```python
from build123d import *

# Parameters (mm, degrees)
F0_W     = 170
F0_H     = 30
F1_DEPTH = 13
F3_DEPTH = 28
F4_W     = 110
F4_H     = 2
F5_DEPTH = 5
F6_SIZE  = 10
F7_R     = 5
F8_SIZE  = 1
F9_R     = 2


with BuildPart() as f1:
    # F0 (on Front) → F1 (new body)
    with BuildSketch(Plane.XZ):
        with Locations((0, 15)):
            Rectangle(F0_W, F0_H)
    extrude(amount=F1_DEPTH)

    # F2 (on face) → F3 (cut)
    with BuildSketch(Plane.XY.offset(30)):
        Polygon((-55, -2), (-71, -2), (-71, -12), (-65, -12), (-65, -13), (65, -13), (65, -12), (71, -12), (71, -2), (55, -2), (55, 0), (-55, 0), align=None)
    extrude(amount=-F3_DEPTH, mode=Mode.SUBTRACT)

    # F4 (on face) → F5 (join)
    with BuildSketch(Plane.XY.offset(2)):
        with Locations((0, -1)):
            Rectangle(F4_W, F4_H)
    extrude(amount=F5_DEPTH)

    # F6
    f6_edges = [f1.edges().sort_by_distance(p)[0] for p in [
        (85, -6.5, 0),
        (-85, -6.5, 0),
    ]]
    chamfer(f6_edges, length=F6_SIZE)

    # F7
    f7_edges = [f1.edges().sort_by_distance(p)[0] for p in [
        (-71, -7, 2),
        (71, -7, 2),
    ]]
    fillet(f7_edges, radius=F7_R)

    # F8
    f8_edges = [f1.edges().sort_by_distance(p)[0] for p in [
        (0, -13, 0),
        (0, 0, 0),
    ]]
    chamfer(f8_edges, length=F8_SIZE)

    # F9
    f9_edges = [f1.edges().sort_by_distance(p)[0] for p in [
        (-85, -6.5, 10),
        (-85, -6.5, 30),
        (-71, -7, 30),
        (71, -7, 30),
        (85, -6.5, 30),
        (85, -6.5, 10),
        (55, -1, 7),
        (55, -1, 30),
        (65, -12.5, 2),
        (65, -12.5, 30),
        (-55, -1, 30),
        (-55, -1, 7),
        (-65, -12.5, 2),
        (-65, -12.5, 30),
        (85, 0, 20),
        (80.5, 0, 5.5),
        (80.5, -13, 5.5),
        (85, -13, 20),
        (-85, 0, 20),
        (-80.5, 0, 5.5),
        (-85, -13, 20),
        (-80.5, -13, 5.5),
    ]]
    fillet(f9_edges, radius=F9_R)


solid = f1.part
```
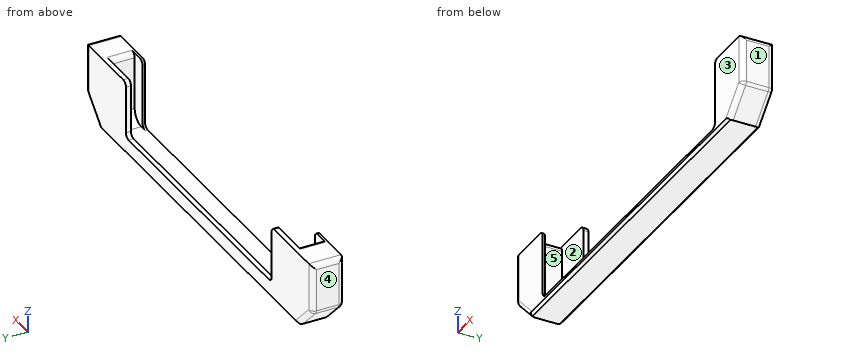
Geometry check sheet. Reference: the model listing, model coordinates, mm. Face numbers are marked on the shaded views. A direction names the side the tool comes from. Coordinates: 2 decimals unless noted, no trailing zeros. Write each loop counter-clockwise with the first axis right and the second up, starting at its lowest first coordinate (ties: lowest second). Pieces come first, ordered by that corner, then holes. Notation, with made-up numbers: M -10,51.5 L 7,51.5 A20 ccw 7,82.5 Z; hole C 45,70 d3. An arc over 180 degrees is marked long. One line per item, written item: value. Start each with the question number.
(1) Sectioned sample at D-D, the plane x = 60.5. Enter the section's corners in (y, z), and give its area (3 significant figures).
(2) Depth check by flat-ended pin: pin 1 (10 mm diameter, centred on x = 55.5, z = 13, fed in from +Y); pin 2 (1.6 mm diameter, centred on x = -6.5, y = -1.5, fed in from +Z); pin 3 (0.6 mm diameter, centred on y = -0.5, z = 14.5, fed in from -X); pin 4 (2 mm diameter, centred on y = -7, z = 7.5, fed in from +X). Enter the tip coordinate at first touch or a pass-through.
(3) Release check for a two-part mould opening along X. For the marked faces 1, 2 and 3 record: released by +X, released by -X, zero draft, split by the parting line, or undercut.
(4) Sectioned sample at C-C, the plane y = -8.75. Enter the section's corners in (x, z), and give its area (3 significant figures).
(5) Scan lines: line 1 along X through (y, z) = (-9.75, 26); line 2 along Z through (x, y) = (9.5, -8); line 3 along X through (y, z) = (-5.25, 6.5). Record each from-to range of solid material in increasing order. Write a range as [from, to].
(6) Tool access check on the marked faces 4 and 5. Record the directions out of +Z, -Z, +X, -X, +Y, -Y that give a thin tool (end or side, any length) a straight path to the whole face; none if there is none.
(7) Sectioned sample at B-B, the plane x = 27. Enter the section's corners in (y, z).
(8) Sectioned sample at A-A, the plane z = 24. Enter the section's corners in (x, y), and give its area (3 significant figures).
Filled sheet:
1. outline: M -13,1 L -12,0 L -1,0 L 0,1 L 0,30 L -2,30 L -2,2 L -13,2 Z
1. area: 81.0 mm²
2. pin 1: y = 0
2. pin 2: z = 7
2. pin 3: x = -84.6
2. pin 4: x = 83.5
3. face 1: released by +X
3. face 2: undercut
3. face 3: zero draft
4. outline: M -85,10.83 A2 ccw -84.41,9.41 L -75,0 L 75,0 L 84.41,9.41 A2 ccw 85,10.83 L 85,28 A2 ccw 83,30 L 73,30 A2 ccw 71,28 L 71,7 A5 cw 66,2 L -66,2 A5 cw -71,7 L -71,28 A2 ccw -73,30 L -83,30 A2 ccw -85,28 Z
4. area: 1,030 mm²
5. line 1: [-85, -71], [71, 85]
5. line 2: [0, 2]
5. line 3: [-81.5, -70.97], [70.97, 81.5]
6. face 4: +Z, -Z, -X, +Y, -Y
6. face 5: +Z
7. outline: M -13,1 L -12,0 L -1,0 L 0,1 L 0,7 L -2,7 L -2,2 L -13,2 Z
8. outline: M -85,-11 A2 ccw -83,-13 L -65,-13 L -65,-12 L -71,-12 L -71,-2 L -55,-2 L -55,0 L -83,0 A2 ccw -85,-2 Z; M 55,-2 L 71,-2 L 71,-12 L 65,-12 L 65,-13 L 83,-13 A2 ccw 85,-11 L 85,-2 A2 ccw 83,0 L 55,0 Z
8. area: 437 mm²
